from build123d import *

# Parameters (mm, degrees)
F0_W     = 1828.8
F0_H     = 914.4
F1_DEPTH = 635
F3_DEPTH = 558.8


with BuildPart() as f1:
    # F0 (on Top) → F1 (new body)
    with BuildSketch(Plane.XY):
        Rectangle(F0_W, F0_H)
    extrude(amount=F1_DEPTH)

    # F2 (on face) → F3 (cut)
    with BuildSketch(Plane(origin=(0, 0, 0), x_dir=(1, 0, 0), z_dir=(0, 0, -1))):
        Polygon((838.2, 457.2), (-838.2, 457.2), (-838.2, 381), (-914.4, 381), (-914.4, -381), (-838.2, -381), (-838.2, -457.2), (838.2, -457.2), (838.2, -381), (914.4, -381), (914.4, 381), (838.2, 381), align=None)
    extrude(amount=-F3_DEPTH, mode=Mode.SUBTRACT)


solid = f1.part
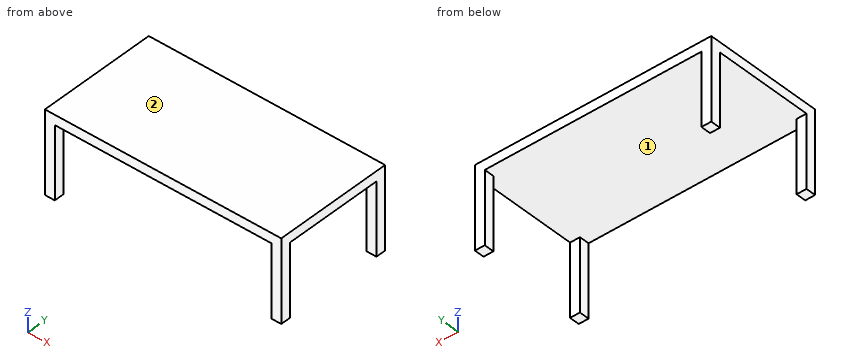
Input: part model. Units: mm. Frame: model coordinates. Face numbers are marked on the shaded views. Give positions to 0.01 mm unless a question says otherwise; leave off trailing zeros. Order: outer loops, then holes, each group sorted by start corner. A loop starts at its lowest first (then second) coordinate and runs counter-clockwise, first axis right, second up.
Q1. Section A-A on z = 223. Output: boundary loops of the cut face in (x, y), and give its area (3 significant figures).
Checked values:
outline: (-914.4, -457.2) - (-838.2, -457.2) - (-838.2, -381) - (-914.4, -381) - close; (-914.4, 381) - (-838.2, 381) - (-838.2, 457.2) - (-914.4, 457.2) - close; (838.2, -457.2) - (914.4, -457.2) - (914.4, -381) - (838.2, -381) - close; (838.2, 381) - (914.4, 381) - (914.4, 457.2) - (838.2, 457.2) - close
area: 23,200 mm2
Q2. Draft query along X for the marked faces 1 and 2. Return one class per face: +X half, -X half, draft (parallel to the pull), parting line (faces both ways), or undercut.
Checked values:
face 1: undercut
face 2: draft
Q3. Section B-B on y = -97. Output: boundary loops of the cut face in (x, z), and give its area (3 significant figures).
Checked values:
outline: (-914.4, 558.8) - (914.4, 558.8) - (914.4, 635) - (-914.4, 635) - close
area: 139,000 mm2
Q4. Ray query, probe 1 along Z at (x, y) = (-610.5, 414). Return the intervals inside material, ascending.
Checked values:
probe 1: z = 558.8 to 635
Q5. Section C-C on x = -597.5. Output: boundary loops of the cut face in (y, z).
Checked values:
outline: (-457.2, 558.8) - (457.2, 558.8) - (457.2, 635) - (-457.2, 635) - close
Q6. Contact query for a flat-ended pin moving along its axis: pin 1 Ø1 at (x, y) = (-578, 278.5) entering from -Z. Output: stop coordinate, or through.
Checked values:
pin 1: stops at z = 558.8
